```python
from build123d import *

# Parameters (mm, degrees)
F0_R     = 2.5
F0_W     = 2
F0_H     = 11
F1_DEPTH = 2
F2_DEPTH = 5
F3_R     = 4
F4_DEPTH = 5
F5_R     = 20
F5_R_2   = 4
F6_DEPTH = 10
F7_R     = 5
F8_R     = 2


with BuildPart() as f1:
    # F0 (on Front) → F1 (new body)
    with BuildSketch(Plane.XZ):
        with BuildLine():
            Line((5, -77.5), (5, 77.5))
            ThreePointArc((5, 77.5), (3.535534, 81.035534), (0, 82.5))
            ThreePointArc((0, 82.5), (-3.535534, 81.035534), (-5, 77.5))
            Line((-5, 77.5), (-5, -77.5))
            ThreePointArc((-5, -77.5), (-3.535534, -81.035534), (0, -82.5))
            ThreePointArc((0, -82.5), (3.535534, -81.035534), (5, -77.5))
        make_face()
        with Locations((0, -67.5)):
            Circle(F0_R, mode=Mode.SUBTRACT)
        with Locations((0, -57.5)):
            Circle(F0_R, mode=Mode.SUBTRACT)
        with Locations((0, -17.5)):
            Circle(F0_R, mode=Mode.SUBTRACT)
        with Locations((0, -7.5)):
            Circle(F0_R, mode=Mode.SUBTRACT)
        with Locations((0, 72)):
            Rectangle(F0_W, F0_H, mode=Mode.SUBTRACT)
        with Locations((0, -7.5)):
            Circle(F0_R)
        with Locations((0, -17.5)):
            Circle(F0_R)
        with Locations((0, -57.5)):
            Circle(F0_R)
        with Locations((0, -67.5)):
            Circle(F0_R)
    extrude(amount=F1_DEPTH)

    # F0 (on Front) → F2 (join)
    with BuildSketch(Plane.XZ):
        with Locations((0, -7.5)):
            Circle(F0_R)
        with Locations((0, -57.5)):
            Circle(F0_R)
    extrude(amount=-F2_DEPTH)

    # F3 (on face) → F4 (join)
    with BuildSketch(Plane.XZ.offset(2)):
        with Locations((0, -37.5)):
            Circle(F3_R)
    extrude(amount=F4_DEPTH)

    # F5 (on face) → F6 (join)
    with BuildSketch(Plane.XZ.offset(7)):
        with Locations((0, -37.5)):
            Circle(F5_R)
        with Locations((0, -37.5)):
            Circle(F5_R_2)
    extrude(amount=F6_DEPTH)

    # F7
    f7_edges = [f1.edges().sort_by_distance(p)[0] for p in [
        (-20, -17, -37.5),
    ]]
    fillet(f7_edges, radius=F7_R)

    # F8
    f8_edges = [f1.edges().sort_by_distance(p)[0] for p in [
        (-4, -7, -37.5),
        (-20, -7, -37.5),
    ]]
    fillet(f8_edges, radius=F8_R)


solid = f1.part
```
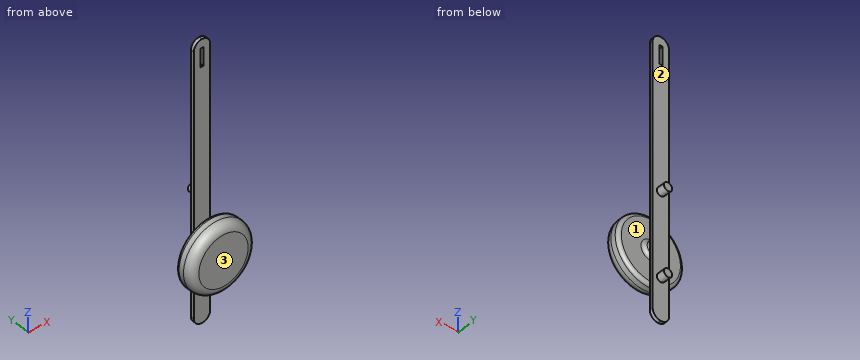
Verification items for the finished model (mm, model axes). Face numbers are marked on the shaded views. Give positions to 0.01 mm unless a question says otherwise; leave off trailing zeros. Loops run counter-clockwise (first coordinate to the right, second up) from the corner with the lowest first, then second, coordinate; pieces in that order, holes last.
1. Section check C-C, the plane y = -13.75. Enter the section's corners in (x, z).
2. Section check B-B, the plane z = 20. Enter the section's corners in (x, y).
3. Section check A-A, the plane z = -37.5. Enter the section's corners in (x, y).
4. Mould release check, pull along Y, two halves, no side actions. Record for the marked faces 1, 2 and 3: released by +Y, released by -Y, zero draft, split by the parting line, or undercut.
5. Thickness scan on line 1 (X direction, y = -0.75, z = 46); line 2 (Y direction, x = 0, z = 14.5); line 3 (Y direction, x = -7.5, z = -31). Record the ranges inside material, lowest first.
6. Go/stop test with flat-tipped pins: pin 1 Ø5 at (y, z) = (-0.5, 30.5) entering from +X; pin 2 Ø1 at (y, z) = (-1.5, 70.5) entering from -X; pin 3 Ø11 at (x, z) = (0.5, 3.5) entering from -Y. Record where each tip stops, or that it passes through.
Geometry says:
1. outline: circle Ø39.37 at (0, -37.5)
2. outline: (-5, -2) - (5, -2) - (5, 0) - (-5, 0) - close
3. outline: (-20, -12) arc R5 ccw to (-15, -17) - (15, -17) arc R5 ccw to (20, -12) - (20, -9) arc R2 ccw to (18, -7) - (6, -7) arc R2 cw to (4, -5) - (4, -2) - (5, -2) - (5, 0) - (-5, 0) - (-5, -2) - (-4, -2) - (-4, -5) arc R2 cw to (-6, -7) - (-18, -7) arc R2 ccw to (-20, -9) - close
4. face 1: undercut
4. face 2: released by +Y
4. face 3: released by -Y
5. line 1: x = -5 to 5
5. line 2: y = -2 to 0
5. line 3: y = -17 to -7
6. pin 1: stops at x = 5
6. pin 2: stops at x = -5
6. pin 3: stops at y = -2
